from build123d import *

# Parameters (mm, degrees)
SKETCH093_R     = 1.75
SKETCH093_R_2   = 2.75
SKETCH093_R_3   = 11.5
PAD032_DEPTH    = 6.35
SKETCH094_R     = 3
POCKET027_DEPTH = 3


with BuildPart() as part:
    # Sketch093 → Pad032 (new body)
    with BuildSketch(Plane.XY):
        with BuildLine():
            Line((-34.637223, 4.338048), (-20.137223, 19.838048))
            ThreePointArc((-15.5, 21.85), (-18.027439, 21.325337), (-20.137223, 19.838048))
            Line((-15.5, 21.85), (15.5, 21.85))
            ThreePointArc((20.137223, 19.838048), (18.027439, 21.325337), (15.5, 21.85))
            Line((20.137223, 19.838048), (34.637223, 4.338048))
            ThreePointArc((34.637223, -4.338048), (36.35, 0), (34.637223, 4.338048))
            Line((34.637223, -4.338048), (20.137223, -19.838048))
            ThreePointArc((15.5, -21.85), (18.027439, -21.325337), (20.137223, -19.838048))
            Line((15.5, -21.85), (-15.5, -21.85))
            ThreePointArc((-20.137223, -19.838048), (-18.027439, -21.325337), (-15.5, -21.85))
            Line((-20.137223, -19.838048), (-34.637223, -4.338048))
            ThreePointArc((-34.637223, 4.338048), (-36.35, 0), (-34.637223, -4.338048))
        make_face()
        with Locations((-15.5, 15.5)):
            Circle(SKETCH093_R, mode=Mode.SUBTRACT)
        with Locations((15.5, 15.5)):
            Circle(SKETCH093_R, mode=Mode.SUBTRACT)
        with Locations((15.5, -15.5)):
            Circle(SKETCH093_R, mode=Mode.SUBTRACT)
        with Locations((-15.5, -15.5)):
            Circle(SKETCH093_R, mode=Mode.SUBTRACT)
        with Locations((-30, 0)):
            Circle(SKETCH093_R_2, mode=Mode.SUBTRACT)
        with Locations((30, 0)):
            Circle(SKETCH093_R_2, mode=Mode.SUBTRACT)
        Circle(SKETCH093_R_3, mode=Mode.SUBTRACT)
    extrude(amount=PAD032_DEPTH)

    # Sketch094 → Pocket027 (cut)
    with BuildSketch(Plane.XY):
        with Locations((-15.5, 15.5)):
            Circle(SKETCH094_R)
        with Locations((15.5, 15.5)):
            Circle(SKETCH094_R)
        with Locations((15.5, -15.5)):
            Circle(SKETCH094_R)
        with Locations((-15.5, -15.5)):
            Circle(SKETCH094_R)
    extrude(amount=POCKET027_DEPTH, mode=Mode.SUBTRACT)


solid = part.part
Geometry check sheet. Reference: the model listing, model coordinates, mm. A direction names the side the tool comes from. Give positions to 0.01 mm unless a question says otherwise; leave off trailing zeros. Write each loop counter-clockwise with the first axis right and the second up, starting at its lowest first coordinate (ties: lowest second). Pieces come first, ordered by that corner, then holes. Notation, with made-up numbers: M 60.5,80.25 L 107.5,80.25 A16 cw 107.5,95.25 Z; hole C -36.5,10 d2. An arc over 180 degrees is marked long. Answer as CSV lines item,"result". Start each with the question number.
Q1. Section check D-D, the plane y = 6. Record the cut outline in (x, z), then the cut area to 3 significant figures.
Q2. Section check C-C, the plane x = 0. Record the cut outline in (y, z).
Q3. Section check A-A, the plane y = 0. Record the cut outline in (x, z).
Q4. Tool access check on faces 1 (the face through (-16.15, -18.43, 1.48)), 2 (the face through (0, 21.85, 3)). Record the directions out of +Z, -Z, +X, -X, +Y, -Y that give a thin tool (end or side, any length) a straight path to the whole face; none if there is none.
Q5. Material ranges on L1, parallel to Y at x = 15.5, z = 2.1; L2, parallel to Y at x = -15.5, z = 4.15; L3, parallel to X at y = -15.5, z = 4.7, recorded low to high.
Q6. Release check for a two-part mould opening along X. For faces 3 (the face through (9, 10, 6.35)), 4 (the face through (-27.49, 11.98, 3.13)), 5 (the face through (15.272, -13.765, 4.652)) record: pulls with the +X half, pulls with the -X half, needs draft (parallel to the pull), parting line crosses it, or undercut.
Q7. Go/stop test with flat-tipped pins: pin 1 (6 mm diameter, centred on x = -28.5, y = 16, fed in from -Z); pin 2 (4.5 mm diameter, centred on x = -15.5, y = 15.5, fed in from -Z). Record where each tip stops, or that it passes through.
Q8. Section check B-B, the plane z = 0.75. Record the cut outline in (x, y), then the cut area to 3 significant figures.
Geometry says:
1,outline,"M -33.08,0 L -9.81,0 L -9.81,6.35 L -33.08,6.35 Z; M 9.81,0 L 33.08,0 L 33.08,6.35 L 9.81,6.35 Z"
1,area,"296 mm^2"
2,outline,"M -21.85,0 L -11.5,0 L -11.5,6.35 L -21.85,6.35 Z; M 11.5,0 L 21.85,0 L 21.85,6.35 L 11.5,6.35 Z"
3,outline,"M -36.35,0 L -32.75,0 L -32.75,6.35 L -36.35,6.35 Z; M -27.25,0 L -11.5,0 L -11.5,6.35 L -27.25,6.35 Z; M 11.5,0 L 27.25,0 L 27.25,6.35 L 11.5,6.35 Z; M 32.75,0 L 36.35,0 L 36.35,6.35 L 32.75,6.35 Z"
4,face 1,"-Z"
4,face 2,"+Z, -Z, +X, -X, +Y"
5,L1,"-21.85 to -18.5, -12.5 to 12.5, 18.5 to 21.85"
5,L2,"-21.85 to -17.25, -13.75 to 13.75, 17.25 to 21.85"
5,L3,"-24.2 to -17.25, -13.75 to 13.75, 17.25 to 24.2"
6,face 3,"needs draft"
6,face 4,"pulls with the -X half"
6,face 5,"undercut"
7,pin 1,"through"
7,pin 2,"z = 3"
8,outline,"M -34.64,-4.34 L -20.14,-19.84 A6.35 ccw -15.5,-21.85 L 15.5,-21.85 A6.35 ccw 20.14,-19.84 L 34.64,-4.34 A6.35 ccw 34.64,4.34 L 20.14,19.84 A6.35 ccw 15.5,21.85 L -15.5,21.85 A6.35 ccw -20.14,19.84 L -34.64,4.34 A6.35 ccw Z; hole C -30,0 d5.5; hole C -15.5,-15.5 d6; hole C -15.5,15.5 d6; hole C 0,0 d23; hole C 15.5,-15.5 d6; hole C 15.5,15.5 d6; hole C 30,0 d5.5"
8,area,"1,890 mm^2"
